The drawing under review shows one solid part. Ordinate dimensions are in mm from its lowest x, y, z. A direction names the side the tool comes from. Coordinates: 2 decimals unless noted, no trailing zeros. Write each loop counter-clockwise with the first axis right and the second up, starting at its lowest first coordinate (ties: lowest second). Pieces come first, ordered by that corner, then holes.
Q1. Machinability: for the marked faces 1, 2 and 3, which of the approach directions +Z, -Z, +X, -X, +Y, -Y give a long, thin tool a straight path to every point of the face, cutting with its end or side? Answer none if there is none.
Q2. Take a section at A-A (x = 6.35). Give the boundary of the cut face in (y, z), and give its area (3 significant figures).
Q3. Take a section at C-C (y = 22). Give the boundary of the cut face in (x, z), and give its area (3 significant figures).
Q4. Insertion check: pin 1 (5 mm diameter, centred on x = 2, z = 2, fed in from +Y); pin 2 (1.5 mm diameter, centred on x = 6, z = 11, fed in from -Y); pin 3 (2 mm diameter, centred on x = 10, y = 15, fed in from +Z). Each pin has a flat end and moves straight along its axis. Give the tip position at first contact, or say it passes through.
Q5. Take a section at B-B (z = 6.35). Give the boundary of the cut face in (x, y).
Q6. For probe 1 along Y at (x, z) = (10, 3.25); probe 2 along X at (y, z) = (6, 6.5); probe 3 along Z at (x, y) = (6.5, 22.5), list the stretches that pass through material, from the lowest coordinate up.
Q7. Take a section at D-D (y = 28). Give the boundary of the cut face in (x, z), and give its area (3 significant figures).
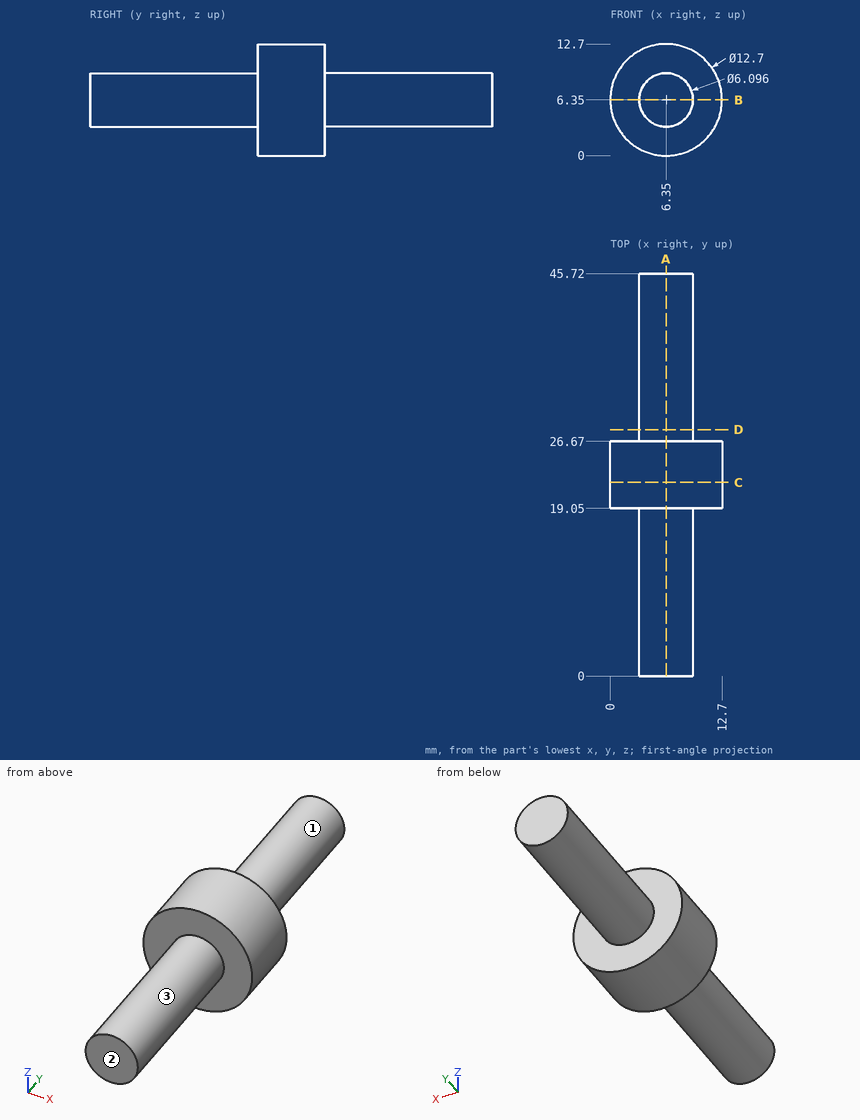
Response:
1. face 1: +Y
1. face 2: +Z, -Z, +X, -X, -Y
1. face 3: -Y
2. outline: (0, 3.3) - (19.05, 3.3) - (19.05, 0) - (26.67, 0) - (26.67, 3.3) - (45.72, 3.3) - (45.72, 9.4) - (26.67, 9.4) - (26.67, 12.7) - (19.05, 12.7) - (19.05, 9.4) - (0, 9.4) - close
2. area: 329 mm2
3. outline: circle Ø12.7 at (6.35, 6.35)
3. area: 127 mm2
4. pin 1: stops at y = 26.67
4. pin 2: stops at y = 19.05
4. pin 3: stops at z = 7.86
5. outline: (0, 19.05) - (3.3, 19.05) - (3.3, 0) - (9.4, 0) - (9.4, 19.05) - (12.7, 19.05) - (12.7, 26.67) - (9.4, 26.67) - (9.4, 45.72) - (3.3, 45.72) - (3.3, 26.67) - (0, 26.67) - close
6. probe 1: y = 19.05 to 26.67
6. probe 2: x = 3.31 to 9.39
6. probe 3: z = 0 to 12.7
7. outline: circle Ø6.1 at (6.35, 6.35)
7. area: 29.2 mm2
